For this review, take the finished solid that the model builds, in its own axes (mm). Coordinates: 2 decimals unless noted, no trailing zeros. Order: outer loops, then holes, each group sorted by start corner. A loop starts at its lowest first (then second) coordinate and runs counter-clockwise, first axis right, second up. Notation, with made-up numbers: (-20.5, 88) -> (34.5, 88) arc R35 cw to (34.5, 124) -> close; hole circle Ø5 at (-6, 80.5). An arc over 180 degrees is marked (long way). Answer as a JSON object with one key per item and string values. Group by question number.
1) Add section B-B, the plane z = 0. Write out the cut boundary in (x, y).
2) For pin 1 (6.5 mm diameter, centred on y = 0, z = 0, fed in from -X), flat-tipped, find the tip position at first contact; note if it passes through.
3) Add section A-A, the plane y = -25.4. Write out the cut boundary in (x, z), then the cut area to 3 significant figures.
4) Add section C-C, the plane x = 1.2. Write out the cut boundary in (y, z).
5) Add section D-D, the plane z = 4.25. Write out the cut boundary in (x, y).
6) Wall thickness on L1, parallel to Z at x = 1.1, y = -25.4; L2, parallel to Y at x = 0.6, z = 0.5; L3, parallel to Y at x = 0.6, z = 0: over which ranges is each line inside the solid? List them lowest first.
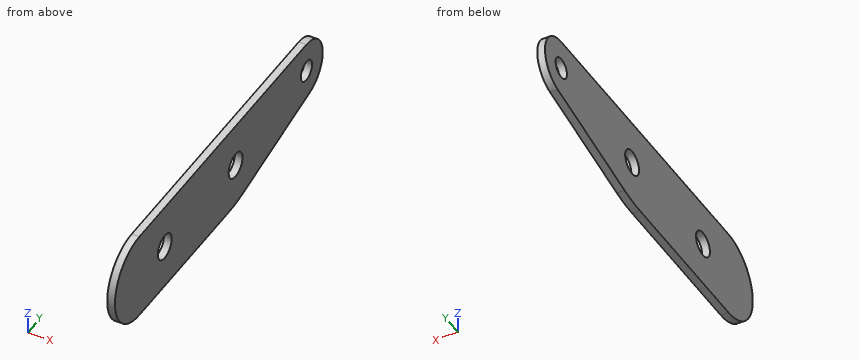
from build123d import *

# Parameters (mm, degrees)
SKETCH1_R           = 2.4892
SKETCH1_R_2         = 2.032
BOSS_EXTRUDE1_DEPTH = 1.524
FILLET1_R           = 25.4


with BuildPart() as part:
    # Sketch1 → Boss-Extrude1 (new body)
    with BuildSketch(Plane(origin=(0, 0, 0), x_dir=(0, 0, -1), z_dir=(1, 0, 0))):
        with BuildLine():
            Line((8.763, -34.506990432), (8.763, 0))
            Line((8.763, 0), (2.779382525, 26.678515962))
            ThreePointArc((2.779382525, 26.678515962), (-3.564167663, 31.206487695), (-8.763, 25.4))
            Line((-8.763, 25.4), (-8.763, -34.506990432))
            ThreePointArc((-8.763, -34.506990432), (0, -43.269990432), (8.763, -34.506990432))
        make_face()
        with Locations(Location((0, 0, 0), (0, 0, 180))):
            Circle(SKETCH1_R, mode=Mode.SUBTRACT)
        with Locations(Location((0, -25.4, 0), (0, 0, 180))):
            Circle(SKETCH1_R, mode=Mode.SUBTRACT)
        with Locations(Location((-2.921, 25.4, 0), (0, 0, 180))):
            Circle(SKETCH1_R_2, mode=Mode.SUBTRACT)
    extrude(amount=BOSS_EXTRUDE1_DEPTH)

    # Fillet1
    fillet1_edges = [part.edges().sort_by_distance(p)[0] for p in [
        (0.762, 0, -8.763),
    ]]
    fillet(fillet1_edges, radius=FILLET1_R)


solid = part.part
Output values:
{
 "1": {"outline": "(0, -43.27) -> (1.52, -43.27) -> (1.52, -27.89) -> (0, -27.89) -> close; (0, -22.91) -> (1.52, -22.91) -> (1.52, -2.49) -> (0, -2.49) -> close; (0, 2.49) -> (1.52, 2.49) -> (1.52, 30.46) -> (0, 30.46) -> close"},
 "2": {"pin 1": "stops at x = 0"},
 "3": {"outline": "(0, -8.76) -> (1.52, -8.76) -> (1.52, -2.49) -> (0, -2.49) -> close; (0, 2.49) -> (1.52, 2.49) -> (1.52, 8.76) -> (0, 8.76) -> close", "area": "19.1 mm²"},
 "4": {"outline": "(-34.51, -8.76) -> (-2.81, -8.76) arc R25.4 ccw to (2.75, -8.15) -> (26.68, -2.78) arc R5.84 ccw to (25.4, 8.76) -> (-34.51, 8.76) arc R8.76 ccw to start; hole circle Ø4.98 at (-25.4, 0); hole circle Ø4.98 at (0, 0); hole circle Ø4.06 at (25.4, 2.92)"},
 "5": {"outline": "(0, -42.17) -> (1.52, -42.17) -> (1.52, 23.86) -> (0, 23.86) -> close; (0, 26.94) -> (1.52, 26.94) -> (1.52, 31.09) -> (0, 31.09) -> close"},
 "6": {"L1": "z = -8.76 to -2.49, 2.49 to 8.76", "L2": "y = -43.26 to -27.84, -22.96 to -2.44, 2.44 to 30.72", "L3": "y = -43.27 to -27.89, -22.91 to -2.49, 2.49 to 30.46"}
}
